Autodesk Inventor part; units mm, degrees
ref_plane "YZ Plane" through (0, 0, 0) normal (1, 0, 0) x (0, 1, 0)
ref_plane "XZ Plane" through (0, 0, 0) normal (0, 1, 0) x (-1, 0, 0)
ref_plane "XY Plane" through (0, 0, 0) normal (0, 0, 1) x (1, 0, 0)
sketch "Sketch1" plane through (0, 0, 0) normal (0, 0, 1) x (1, 0, 0)
  line L0 (-45, -72.5) -> (45, -72.5)
  line L1 (45, -72.5) -> (45, 72.5)
  line L2 (45, 72.5) -> (-45, 72.5)
  line L3 (-45, 72.5) -> (-45, -72.5)
  line L4 (-45, -72.5) -> (45, 72.5) construction
  line L5 (45, -72.5) -> (-45, 72.5) construction
  point P0 (0, 0)
  dimension "d154" = 90
  dimension "d155" = 145
extrude "Plate3" add sketch "Sketch1" along normal blind 3
sketch "Sketch7" plane through (42.8787, 72.5, 2.1213) normal (0.7071068, 0, -0.7071068) x (0, 1, 0)
  line L0 (-145, 0) -> (0, 0)
  line L1 (0, 0) -> (0, 78)
  line L2 (0, 78) -> (-145, 78)
  line L3 (-145, 78) -> (-145, 0)
edge flange "Flange3" height 78 angle 45 thickness 3 bend radius 5 thickness toward (0.7071068, 0, -0.7071068) relief round relief width 3 relief depth 1.5 corner gap 5 corner form 0 edges at (45, 0, 3) (-45, 0, 3) wall of the first edge with corners at (42.8787, -72.5, 2.1213) (42.8787, 72.5, 2.1213) (98.033, 72.5, 57.2756) (98.033, -72.5, 57.2756)
bend "Bend3"
corner "Corner3"
sketch "Sketch8" plane through (0, 0, 3) normal (0, 0, 1) x (1, 0, 0)
  line L0 (23, 62.5) -> (-23, 62.5)
  line L1 (-23, 62.5) -> (-23, -42.5)
  line L2 (-23, -42.5) -> (23, -42.5)
  line L3 (23, -42.5) -> (23, 62.5)
  line L4 (23, 62.5) -> (-23, -42.5) construction
  line L5 (-23, 62.5) -> (23, -42.5) construction
  line L6 (-45, 72.5) -> (41.6863, 72.5)
  line L7 (-41.6863, -72.5) -> (41.6863, -72.5)
  line L8 (23, -72.5) -> (-23, -72.5)
  line L9 (-23, -72.5) -> (-23, -52.5)
  line L10 (-23, -52.5) -> (23, -52.5)
  line L11 (23, -52.5) -> (23, -72.5)
  point P0 (0, 0)
  point P1 (0, 10)
  point P2 (-23, -72.5)
  point P3 (33.1873, -84)
  dimension "d166" = 46
  dimension "d168" = 10
  dimension "d182" = 10
  dimension "d183" = 20
extrude "Cut1" cut sketch "Sketch8" against normal blind 3
sketch "Sketch9" plane through (-97.1543, -72.5, 55.1543) normal (-1, 0, 0) x (0, -1, 0)
  line L0 (-145, 0) -> (0, 0)
  line L1 (0, 0) -> (0, 87)
  line L2 (0, 87) -> (-145, 87)
  line L3 (-145, 87) -> (-145, 0)
edge flange "Flange4" height 87 angle 45 thickness 3 bend radius 5 thickness toward (-1, 0, 0) relief round relief width 3 relief depth 1.5 edges at (-98.033, 0, 57.2756) wall of the first edge with corners at (-97.1543, 72.5, 55.1543) (-97.1543, -72.5, 55.1543) (-97.1543, -72.5, 142.1543) (-97.1543, 72.5, 142.1543)
bend "Bend4"
corner "Corner4"
sketch "Sketch10" plane through (0, 0, 3) normal (0, 0, 1) x (1, 0, 0)
  line L0 (-38.15, 3.5) -> (-34.85, 3.5)
  line L1 (-34.85, 3.5) -> (-34.85, -3.5)
  line L2 (-34.85, -3.5) -> (-38.15, -3.5)
  line L3 (-38.15, -3.5) -> (-38.15, 3.5)
  line L4 (-38.15, 3.5) -> (-34.85, -3.5) construction
  line L5 (-34.85, 3.5) -> (-38.15, -3.5) construction
  line L6 (34.85, 3.5) -> (38.15, 3.5)
  line L7 (38.15, 3.5) -> (38.15, -3.5)
  line L8 (38.15, -3.5) -> (34.85, -3.5)
  line L9 (34.85, -3.5) -> (34.85, 3.5)
  line L10 (34.85, 3.5) -> (38.15, -3.5) construction
  line L11 (38.15, 3.5) -> (34.85, -3.5) construction
  line L12 (0, 0) -> (0, 29.0693)
  line L13 (41.6863, -72.5) -> (23, -72.5)
  point P0 (-36.5, 0)
  point P1 (36.5, 0)
  point P2 (-36.5, 3.5)
  point P3 (36.5, 3.5)
  dimension "d184" = 7
  dimension "d185" = 3.3
  dimension "d186" = 69
  dimension "d187" = 73
extrude "Cut2" cut sketch "Sketch10" against normal blind 3
properties part number "DSB-101 Axis" material "Stainless Steel"
CAD build for the part. Positions are in the model's coordinates, mm. A direction names the side the tool comes from. Round coordinates to 2 decimals unless told otherwise and drop trailing zeros. Write each loop counter-clockwise with the first axis right and the second up, starting at its lowest first coordinate (ties: lowest second). Pieces come first, ordered by that corner, then holes. Notation, with made-up numbers: M -26.5,59 L 3.5,59 A15 cw 3.5,72 Z; hole C 13,-22.75 d8. An arc over 180 degrees is marked long. Use a Markdown table: item, result. Add a question column.
1. Drill centre lines: probe 1 along X at (y, z) = (-8, 83); probe 2 along X at (y, z) = (-33, 58); probe 3 along Z at (x, y) = (-34, -6.5). Where is each one in solid material? Low to high.
2. Slice it at B-B on x = -20. Give the cut face in (y, z), then the cut area to 3 significant figures.
3. Slice it at D-D on x = 30.5. Give the cut face in (y, z), then the cut area to 3 significant figures.
4. Flat gauge pins, fed straight in: P1, Ø3.5, axis at y = -1, z = 2, coming from the -X side; P2, Ø1.5, axis at x = -2, z = 1.5, coming from the -Y side; P3, Ø5, axis at x = -53, y = 32.5, coming from the -Z side; P4, Ø5, axis at y = 33, z = 53.5, coming from the +X side. Where does each tip first touch, or does it go through?
5. 3-axis set-ups, long thin cutter, end or side, ignore diameter. For faces 1 (the face through (-97.154, -1, 100)), 2 (the face through (44.788, 1.015, 0.626)), 3 (the face through (-28, 1, 3)): which of +Z, -Z, +X, -X, +Y, -Y reach the whole face in a straight line?
6. Slice it at C-C on z = 21. Give the cut face in (x, y).
7. Slice it at A-A on y = -60. Give the cut face in (x, z).
8. Pull direction X, two halves, no side cores. Call faces 4 (the face through (-99.562, -1.015, 55.447)), 5 (the face through (71.26, 1.02, 30.5)), 6 (the face through (-28, 1, 0)): released by +X, released by -X, zero draft, split by the parting line, or undercut.
Reply:
| question | item | result |
|---|---|---|
| 1 | probe 1 | x = -100.15 to -97.15 |
| 1 | probe 2 | x = -100.14 to -97.13 |
| 1 | probe 3 | z = 0 to 3 |
| 2 | outline | M -52.5,0 L -42.5,0 L -42.5,3 L -52.5,3 Z; M 62.5,0 L 72.5,0 L 72.5,3 L 62.5,3 Z |
| 2 | area | 60.0 mm^2 |
| 3 | outline | M -72.5,0 L 72.5,0 L 72.5,3 L -72.5,3 Z |
| 3 | area | 435 mm^2 |
| 4 | P1 | stops at x = -48.75 |
| 4 | P2 | stops at y = -52.5 |
| 4 | P3 | stops at z = 5.5 |
| 4 | P4 | stops at x = 100.15 |
| 5 | face 1 | +Z, +X, +Y, -Y |
| 5 | face 2 | -Z, +X, +Y, -Y |
| 5 | face 3 | +Z, +Y, -Y |
| 6 | outline | M -66,-72.5 L -61.76,-72.5 L -61.76,72.5 L -66,72.5 Z; M 61.76,-72.5 L 66,-72.5 L 66,72.5 L 61.76,72.5 Z |
| 7 | outline | M -100.15,58.47 A8 ccw -97.81,52.81 L -47.34,2.34 A8 ccw -41.69,0 L -23,0 L -23,3 L -41.69,3 A5 cw -45.22,4.46 L -95.69,54.93 A5 cw -97.15,58.47 L -97.15,142.15 L -100.15,142.15 Z; M 23,0 L 41.69,0 A8 ccw 47.34,2.34 L 100.15,55.15 L 98.03,57.28 L 45.22,4.46 A5 cw 41.69,3 L 23,3 Z |
| 8 | face 4 | released by -X |
| 8 | face 5 | undercut |
| 8 | face 6 | zero draft |
